Here's how the part is built. I have some questions about the finished solid (model axes, mm). Face numbers are marked on the shaded views. A direction names the side the tool comes from. Coordinates: 2 decimals unless noted, no trailing zeros. Write each loop counter-clockwise with the first axis right and the second up, starting at its lowest first coordinate (ties: lowest second). Pieces come first, ordered by that corner, then holes.
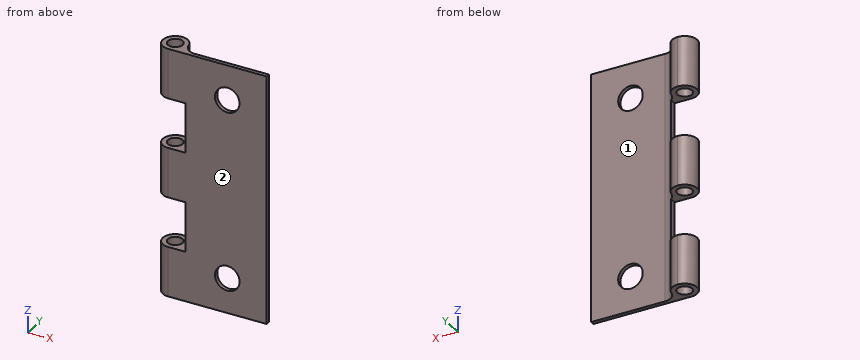
from build123d import *

# Parameters (mm, degrees)
ESBO_O1_R                = 1.5
RESSALTO_EXTRUS_O1_DEPTH = 50
ESBO_O2_R                = 2.5
ESBO_O2_W                = 6
ESBO_O2_H                = 10
CORTE_EXTRUS_O1_DEPTH    = 6


with BuildPart() as part:
    # Esboço1 → Ressalto-extrusão1 (new body)
    with BuildSketch(Plane.XY):
        with BuildLine():
            Line((0, 0), (-20, 0))
            ThreePointArc((-20, 0), (-22.499911314, 2.521057642), (-19.95788621, 4.999645261))
            ThreePointArc((-19.95788621, 4.999645261), (-18.375952887, 4.400650146), (-17.537523452, 2.9315197))
            ThreePointArc((-17.537523452, 2.9315197), (-16.656985327, 1.403588896), (-15, 0.8))
            Line((-15, 0.8), (0, 0.8))
            Line((0, 0.8), (0, 0))
        make_face()
        with Locations((-20, 2.5)):
            Circle(ESBO_O1_R, mode=Mode.SUBTRACT)
    extrude(amount=RESSALTO_EXTRUS_O1_DEPTH)

    # Esboço2 → Corte-extrusão1 (cut, through all)
    with BuildSketch(Plane.XZ):
        with Locations((-8, 43)):
            Circle(ESBO_O2_R)
        with Locations((-8, 7)):
            Circle(ESBO_O2_R)
        with Locations((-19.5, 15)):
            Rectangle(ESBO_O2_W, ESBO_O2_H)
        with Locations((-19.5, 35)):
            Rectangle(ESBO_O2_W, ESBO_O2_H)
    extrude(amount=-CORTE_EXTRUS_O1_DEPTH, mode=Mode.SUBTRACT)


solid = part.part
1. I want a section at C-C (z = 25.5). List the corners of the cut face in (x, y) for me, then the cut area to 3 significant figures.
2. If I drill on line 1 (Z direction, x = -8, y = 0.65); line 2 (Y direction, x = -20, z = 24); line 3 (Y direction, x = -3.5, z = 8.5), over which ranges is the centre line in solid material (lowest first)?
3. I want a section at D-D (z = 33.5). List the corners of the cut face in (x, y) for me.
4. For pin 1 Ø1.5 at (x, z) = (-6.5, 42) entering from +Y; pin 2 Ø1 at (y, z) = (0.5, 33) entering from -X, each with a flat end and sliding along its axis, tell me the tip position at first contact or that it passes through.
5. I want a section at A-A (z = 7). List the corners of the cut face in (x, y) for me, then the cut area to 3 significant figures.
6. On a 3-axis mill with a long thin cutter (end or side, diameter ignored), from which of +Z, -Z, +X, -X, +Y, -Y can I reach the whole of each face in a straight line? I mean the marked faces 1 and 2. Say none if no direction works.
7. I want a section at B-B (x = -8). List the corners of the cut face in (y, z) for me.
Response values:
1. outline: (-20, 0) - (0, 0) - (0, 0.8) - (-15, 0.8) arc R2.58 cw to (-17.54, 2.93) arc R2.5 ccw (long way) to start; hole circle Ø3 at (-20, 2.5)
1. area: 29.2 mm2
2. line 1: z = 0 to 4.5, 9.5 to 40.5, 45.5 to 50
2. line 2: y = 0 to 1, 4 to 5
2. line 3: y = 0 to 0.8
3. outline: (-16.5, 0) - (0, 0) - (0, 0.8) - (-15, 0.8) arc R2.58 cw to (-16.5, 1.28) - close
4. pin 1: stops at y = 0.8
4. pin 2: stops at x = -16.5
5. outline: (-20, 0) - (-10.5, 0) - (-10.5, 0.8) - (-15, 0.8) arc R2.58 cw to (-17.54, 2.93) arc R2.5 ccw (long way) to start; (-5.5, 0) - (0, 0) - (0, 0.8) - (-5.5, 0.8) - close; hole circle Ø3 at (-20, 2.5)
5. area: 25.2 mm2
6. face 1: +Z, -Z, +X, +Y
6. face 2: +Z, -Z, +X, -X, -Y
7. outline: (0, 0) - (0.8, 0) - (0.8, 4.5) - (0, 4.5) - close; (0, 9.5) - (0.8, 9.5) - (0.8, 40.5) - (0, 40.5) - close; (0, 45.5) - (0.8, 45.5) - (0.8, 50) - (0, 50) - close
